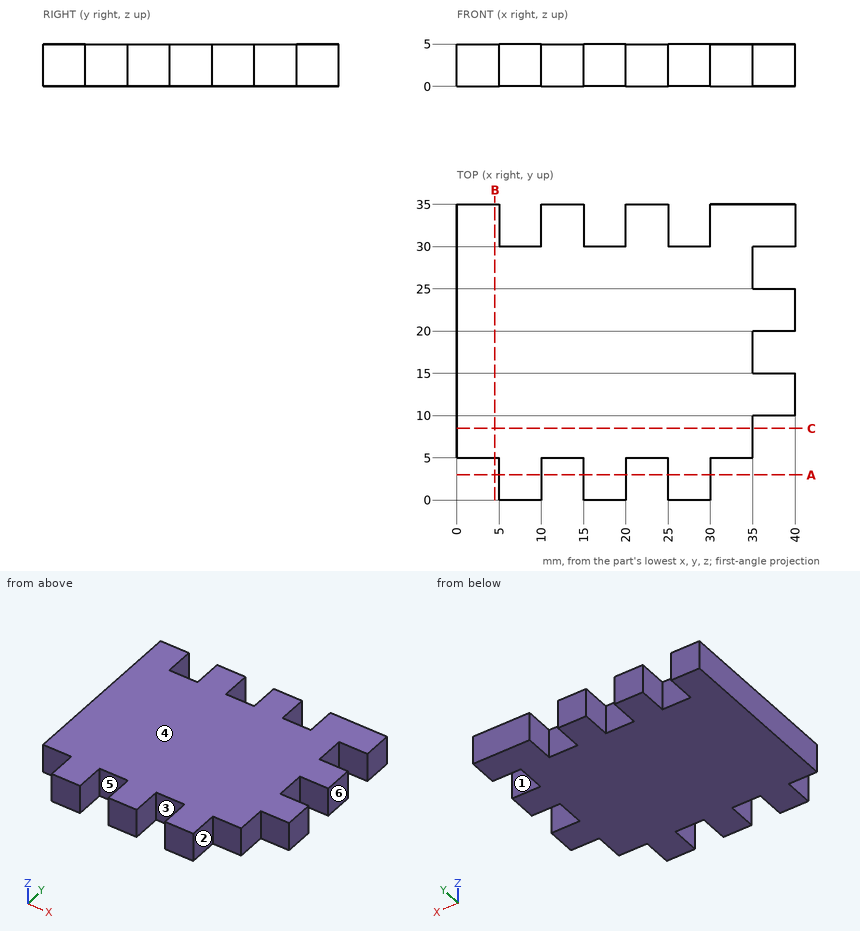
Job drawing, mm, ordinate dimensions from the low corner. One solid piece. A direction names the side the tool comes from. Coordinates: 2 decimals unless noted, no trailing zeros. Order: outer loops, then holes, each group sorted by start corner. A loop starts at its lowest first (then second) coordinate and runs counter-clockwise, first axis right, second up. Notation, with made-up numbers: (-27.75, -32.5) -> (22.25, -32.5) arc R15 cw to (22.25, -10.5) -> close; hole circle Ø6 at (-33.5, 62.25). An arc over 180 degrees is marked (long way). Answer in a Markdown table with one row per item. Add a question column.
Q1. Band-saw the part on C-C, the plane y = 8.5. List the corners of the cut face in (x, z), then the cut area to 3 significant figures.
Q2. Band-saw the part on B-B, the plane x = 4.5. List the corners of the cut face in (y, z).
Q3. Drop flat-ended pins along their axis: pin 1 (2.5 mm diameter, centred on x = 13, z = 3, fed in from -Y); pin 2 (1.5 mm diameter, centred on y = 2.5, z = 1.5, fed in from -X). Give the stop position or say it passes through.
Q4. Band-saw the part on A-A, the plane y = 3. List the corners of the cut face in (x, z).
Q5. Wall check: line 1 along Y through (x, z) = (38, 0.2); line 2 along X through (y, z) = (31.5, 3.25); line 3 along Y through (x, z) = (4, 2.5). Give the ranges that are in metal, low to high. Write a range as [from, to].
Q6. Which spindle directions (+Z, -Z, +X, -X, +Y, -Y) get a long thin tool onto all of the face, cutting with end or side? Do the marked faces 1, 2 and 3. Say none if no direction does.
Q7. Mould opens along X. For the marked faces 4, 5 and 6 say: +X half, -X half, draft (parallel to the pull), parting line (faces both ways), or undercut.
Answers follow:
| question | item | result |
|---|---|---|
| 1 | outline | (0, 0) -> (35, 0) -> (35, 5) -> (0, 5) -> close |
| 1 | area | 175 mm^2 |
| 2 | outline | (5, 0) -> (35, 0) -> (35, 5) -> (5, 5) -> close |
| 3 | pin 1 | y = 5 |
| 3 | pin 2 | x = 5 |
| 4 | outline | (5, 0) -> (10, 0) -> (10, 5) -> (5, 5) -> close; (15, 0) -> (20, 0) -> (20, 5) -> (15, 5) -> close; (25, 0) -> (30, 0) -> (30, 5) -> (25, 5) -> close |
| 5 | line 1 | [10, 15], [20, 25], [30, 35] |
| 5 | line 2 | [0, 5], [10, 15], [20, 25], [30, 40] |
| 5 | line 3 | [5, 35] |
| 6 | face 1 | +Z, -Z, +X |
| 6 | face 2 | +Z, -Z, +X, -Y |
| 6 | face 3 | +Z, -Z, -Y |
| 7 | face 4 | draft |
| 7 | face 5 | undercut |
| 7 | face 6 | +X half |
